```python
from build123d import *

# Parameters (mm, degrees)
F0_W      = 42
F0_H      = 42
F0_R      = 1.5
F0_R_2    = 11
F0_R_3    = 2.5
F1_DEPTH  = 48
F2_DEPTH  = 1.95
F4_DEPTH  = 23.95
F6_DEPTH  = 48.001
F10_DEPTH = 30
F12_R     = 1.5
F13_DEPTH = 43.5


with BuildPart() as f1:
    # F0 (on Top) → F1 (new body)
    with BuildSketch(Plane.XY):
        Rectangle(F0_W, F0_H)
        with Locations((-15.37, -15.37)):
            Circle(F0_R, mode=Mode.SUBTRACT)
        with Locations((15.37, -15.37)):
            Circle(F0_R, mode=Mode.SUBTRACT)
        with Locations((-15.37, 15.37)):
            Circle(F0_R, mode=Mode.SUBTRACT)
        Circle(F0_R_2, mode=Mode.SUBTRACT)
        with Locations((15.37, 15.37)):
            Circle(F0_R, mode=Mode.SUBTRACT)
        Circle(F0_R_2)
        Circle(F0_R_3, mode=Mode.SUBTRACT)
        Circle(F0_R_3)
    extrude(amount=-F1_DEPTH)

    # F0 (on Top) → F2 (join)
    with BuildSketch(Plane.XY):
        Circle(F0_R_2)
        Circle(F0_R_3, mode=Mode.SUBTRACT)
        Circle(F0_R_3)
    extrude(amount=F2_DEPTH)

    # F0 (on Top) → F4 (join, through all)
    with BuildSketch(Plane.XY):
        Circle(F0_R_3)
    extrude(amount=F4_DEPTH)

    # F5 (on face) → F6 (cut, through all)
    with BuildSketch(Plane.XY):
        Polygon((-21, 17.0069894888), (-17.0069894888, 21), (-21, 21), align=None)
        Polygon((-21, -21), (-17.0069894888, -21), (-21, -17.0069894888), align=None)
        Polygon((17.0069894888, 21), (21, 17.0069894888), (21, 21), align=None)
        Polygon((21, -21), (21, -17.0069894888), (17.0069894888, -21), align=None)
    extrude(amount=-F6_DEPTH, mode=Mode.SUBTRACT)

    # F9 (on offset) → F10 (cut, through all)
    with BuildSketch(Plane.XY.offset(-38)):
        Polygon((21, -14.3553390593), (14.3553390593, -21), (17.0069894888, -21), (21, -17.0069894888), align=None)
        Polygon((-21, 17.0069894888), (-21, 14.3553390593), (-14.3553390593, 21), (-17.0069894888, 21), align=None)
        Polygon((-17.0069894888, -21), (-14.3553390593, -21), (-21, -14.3553390593), (-21, -17.0069894888), align=None)
        Polygon((14.3553390593, 21), (21, 14.3553390593), (21, 17.0069894888), (17.0069894888, 21), align=None)
    extrude(amount=F10_DEPTH, mode=Mode.SUBTRACT)

    # F12 (on offset) → F13 (join, through all)
    with BuildSketch(Plane.XY.offset(-4.5)):
        with Locations((-15.37, 15.37)):
            Circle(F12_R)
        with Locations((15.37, 15.37)):
            Circle(F12_R)
        with Locations((15.37, -15.37)):
            Circle(F12_R)
        with Locations((-15.37, -15.37)):
            Circle(F12_R)
    extrude(amount=-F13_DEPTH)


solid = f1.part
```
Check sheet for the modelled part. Datum: model origin and axes. Units: mm. A direction names the side the tool comes from. Round coordinates to 2 decimals unless told otherwise and drop trailing zeros. Order: outer loops, then holes, each group sorted by start corner. A loop starts at its lowest first (then second) coordinate and runs counter-clockwise, first axis right, second up.
1) Mould release check, pull along X, two halves, no side actions. Record for faces 6 (the cylindrical face through (-2.38, -10.74, 0.96)), 7 (the cylindrical face through (16.8, -14.92, -2.22)), 8 (the flat face through (18, -18, -8)): +X half, -X half, draft (parallel to the pull), parting line (faces both ways), or undercut.
2) Tool access check on faces 1 (the flat face through (0, 21, -24)), 2 (the flat face through (-18.976, -19.031, -42.93)), 3 (the flat face through (-10, 10, 0)), 4 (the flat face through (-18, -18, -8)), 5 (the flat face through (-17.724, 17.631, -23.21)). Record the directions out of +Z, -Z, +X, -X, +Y, -Y that give a thin tool (end or side, any length) a straight path to the whole face; none if there is none.
3) Scan lines: line 1 (Z direction, x = -18, y = -19); line 2 (Y direction, x = 15, z = -3); line 3 (Z direction, x = 11.5, y = -2.5). Record each from-to range of solid material in increasing order.
4) Section check A-A (z = -35). Record the boundary of the cut face in (x, y).
5) Go/stop test with flat-tipped pins: pin 1 Ø1.5 at (x, y) = (-15.5, 15.5) entering from +Z; pin 2 Ø3.5 at (x, y) = (16.5, 17.5) entering from +Z. Record where each tip stops, or that it passes through.
6) Section check B-B (y = 0). Record the boundary of the cut face in (x, z).
7) Section check D-D (x = -15.37). Record the boundary of the cut face in (y, z).
Result:
1. face 6: parting line
1. face 7: undercut
1. face 8: draft
2. face 1: +Z, -Z, +X, -X, +Y
2. face 2: +Z, -Z, -X, -Y
2. face 3: +Z
2. face 4: -X, -Y
2. face 5: -X, +Y
3. line 1: z = -48 to -38, -8 to 0
3. line 2: y = -21 to -16.82, -13.92 to 13.92, 16.82 to 21
3. line 3: z = -48 to 0
4. outline: (-21, -14.36) - (-14.36, -21) - (14.36, -21) - (21, -14.36) - (21, 14.36) - (14.36, 21) - (-14.36, 21) - (-21, 14.36) - close
5. pin 1: stops at z = -4.5
5. pin 2: stops at z = 0
6. outline: (-21, -48) - (21, -48) - (21, 0) - (11, 0) - (11, 1.95) - (2.5, 1.95) - (2.5, 23.95) - (-2.5, 23.95) - (-2.5, 1.95) - (-11, 1.95) - (-11, 0) - (-21, 0) - close
7. outline: (-21, -48) - (21, -48) - (21, -38) - (19.99, -38) - (19.99, -8) - (21, -8) - (21, 0) - (16.87, 0) - (16.87, -4.5) - (13.87, -4.5) - (13.87, 0) - (-13.87, 0) - (-13.87, -4.5) - (-16.87, -4.5) - (-16.87, 0) - (-21, 0) - (-21, -8) - (-19.99, -8) - (-19.99, -38) - (-21, -38) - close
